Drawing for the job (mm, zero at the part's lowest x, y, z). A direction names the side the tool comes from. Round coordinates to 2 decimals unless told otherwise and drop trailing zeros. Write each loop counter-clockwise with the first axis right and the second up, starting at its lowest first coordinate (ties: lowest second). Pieces come first, ordered by that corner, then holes.
Item 1: Band-saw the part on A-A, the plane z = 11.1. Write the cut outline in (x, y).
Item 2: Wall check: probe 1 along Y at (x, z) = (2.9, 11.1); probe 2 along Y at (x, z) = (11.75, 11.1); probe 3 along Z at (x, y) = (4, 10.75). Give the ranges that are in metal, low to high.
Item 3: 3-axis set-ups, long thin cutter, end or side, ignore diameter. For the marked faces 4 and 5: which of +Z, -Z, +X, -X, +Y, -Y reach the whole face in a straight line?
Item 4: Drop flat-ended pins along their axis: pin 1 Ø4 at (x, y) = (8.5, 15.5) entering from -Z; pin 2 Ø5 at (x, z) = (7.5, 9) entering from -Y; pin 3 Ø3.5 at (y, z) = (11.1, 3.1) entering from -X; pin 4 Ø2 at (x, y) = (8.5, 8.5) entering from +Z. Give the stop position or say it passes through.
Item 5: Band-saw the part on C-C, the plane y = 3.1. Write the cut outline in (x, z).
Item 6: Mould opens along Y. For the marked faces 1, 2 and 3 say: +Y half, -Y half, draft (parallel to the pull), parting line (faces both ways), or undercut.
Item 7: Band-saw the part on D-D, the plane z = 4.75. Write the cut outline in (x, y), then the cut area to 3 significant figures.
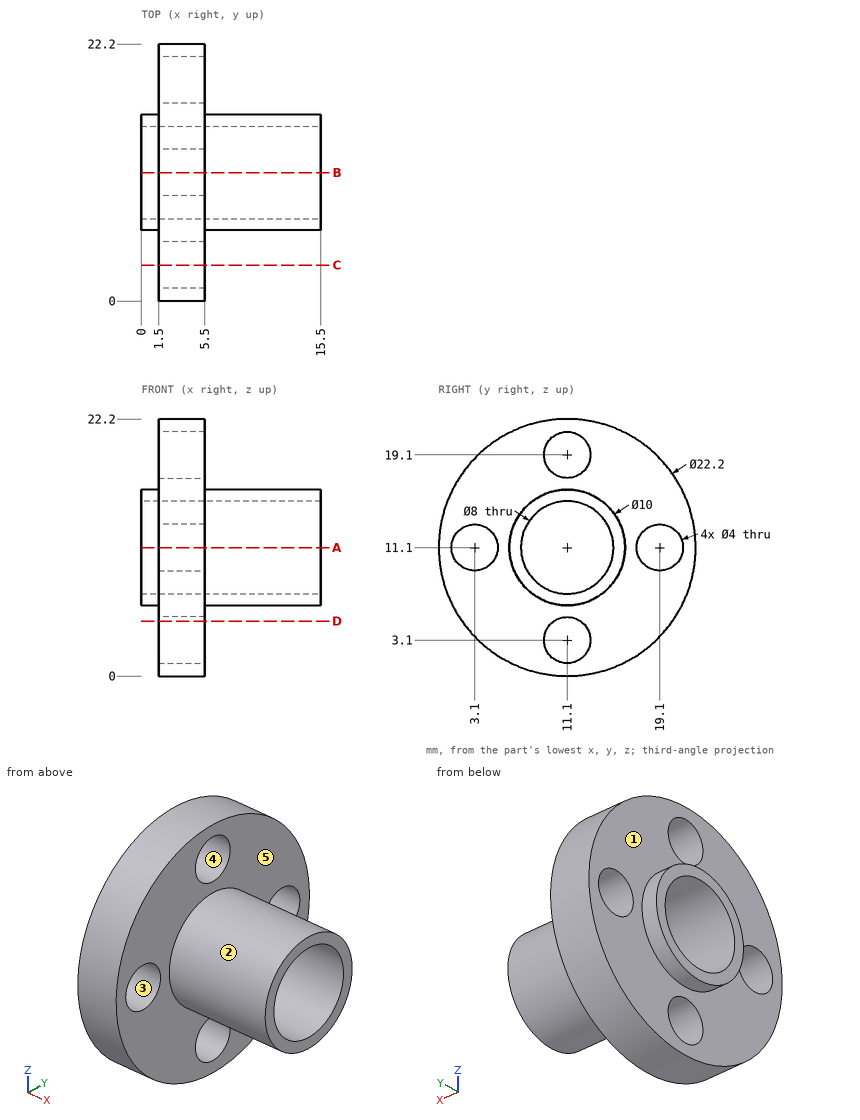
Results:
1. outline: (0, 6.1) - (1.5, 6.1) - (1.5, 5.1) - (5.5, 5.1) - (5.5, 6.1) - (15.5, 6.1) - (15.5, 7.1) - (0, 7.1) - close; (0, 15.1) - (15.5, 15.1) - (15.5, 16.1) - (5.5, 16.1) - (5.5, 17.1) - (1.5, 17.1) - (1.5, 16.1) - (0, 16.1) - close; (1.5, 0) - (5.5, 0) - (5.5, 1.1) - (1.5, 1.1) - close; (1.5, 21.1) - (5.5, 21.1) - (5.5, 22.2) - (1.5, 22.2) - close
2. probe 1: y = 0 to 1.1, 5.1 to 7.1, 15.1 to 17.1, 21.1 to 22.2
2. probe 2: y = 6.1 to 7.1, 15.1 to 16.1
2. probe 3: z = 0.01 to 1.13, 5.07 to 7.12, 15.08 to 17.13, 21.07 to 22.19
3. face 4: +X, -X
3. face 5: +X
4. pin 1: stops at z = 6.71
4. pin 2: stops at y = 0.02
4. pin 3: passes through
4. pin 4: stops at z = 15.84
5. outline: (1.5, 3.41) - (5.5, 3.41) - (5.5, 9.1) - (1.5, 9.1) - close; (1.5, 13.1) - (5.5, 13.1) - (5.5, 18.79) - (1.5, 18.79) - close
6. face 1: draft
6. face 2: parting line
6. face 3: undercut
7. outline: (1.5, 2) - (5.5, 2) - (5.5, 9.97) - (1.5, 9.97) - close; (1.5, 12.23) - (5.5, 12.23) - (5.5, 20.2) - (1.5, 20.2) - close
7. area: 63.8 mm2
